from build123d import *

# Parameters (mm, degrees)
F0_R     = 18.9865
F1_DEPTH = 48.6156
F2_R     = 13.97
F3_DEPTH = 23.9141
F4_R     = 10.16
F5_DEPTH = 24.7025
F6_R     = 11.176
F7_DEPTH = 17.78
F8_R     = 14.224
F9_DEPTH = 17.78
F9_TAPER = 13


with BuildPart() as f1:
    # F0 (on Right) → F1 (new body)
    with BuildSketch(Plane.YZ):
        Circle(F0_R)
    extrude(amount=F1_DEPTH)

    # F2 (on face) → F3 (cut)
    with BuildSketch(Plane(origin=(0, 0, 0), x_dir=(0, -1, 0), z_dir=(-1, 0, 0))):
        Circle(F2_R)
    extrude(amount=-F3_DEPTH, mode=Mode.SUBTRACT)

    # F4 (on face) → F5 (cut, through all)
    with BuildSketch(Plane(origin=(23.9141, 0, 0), x_dir=(0, -1, 0), z_dir=(-1, 0, 0))):
        Circle(F4_R)
    extrude(amount=-F5_DEPTH, mode=Mode.SUBTRACT)

    # F6 (on face) → F7 (cut)
    with BuildSketch(Plane.YZ.offset(48.6156)):
        Circle(F6_R)
    extrude(amount=-F7_DEPTH, mode=Mode.SUBTRACT)

    # F8 (on face) → F9 (cut)
    with BuildSketch(Plane.YZ.offset(48.6156)):
        Circle(F8_R)
    extrude(amount=-F9_DEPTH, taper=F9_TAPER, mode=Mode.SUBTRACT)


solid = f1.part
Design review of the part built by this model. Coordinates are the model's own, in mm. A direction names the side the tool comes from. Coordinates: 2 decimals unless noted, no trailing zeros. Loops run counter-clockwise (first coordinate to the right, second up) from the corner with the lowest first, then second, coordinate; pieces in that order, holes last. Notation, with made-up numbers: (-2, 18) -> (30, 18) arc R15 ccw to (30, 23) -> close; hole circle Ø5 at (18.5, -22.5). An arc over 180 degrees is marked (long way). Use a Markdown table: item, result. Add a question column.
Item 1: The part is to be moulded in two halves that separate along Z. For faces 4 (the flat face through (48.616, 2.7, 14.2)), 5 (the cylindrical face through (23.97, 18.11, 5.7)), 6 (the cylindrical face through (33.16, -8.87, -6.8)), say which applies: +Z half, -Z half, draft (parallel to the pull), parting line (faces both ways), or undercut.
Item 2: Machinability: for faces 1 (the cylindrical face through (11.79, 1.82, 13.85)), 2 (the flat face through (0, -10, 10)), 3 (the flat face through (30.836, -3, -10)), which of the approach directions +Z, -Z, +X, -X, +Y, -Y give a long, thin tool a straight path to every point of the face, cutting with its end or side? Answer none if there is none.
Item 3: We need section D-D, the plane x = 38. Write out the cut boundary in (y, z), and give its area (3 significant figures).
Item 4: Wall thickness on L1, parallel to Z at x = 26, y = -0.5; L2, parallel to Z at x = 12, y = 0; L3, parallel to Y at x = 44, z = 11: over which ranges is each line inside the solid? List them lowest first. Write a range as from..to.
Item 5: We need section B-B, the plane x = 8. Write out the cut boundary in (y, z), and give its area (3 significant figures).
Item 6: We need section A-A, the plane y = 0. Write out the cut boundary in (x, z), and give its area (3 significant figures).
Item 7: We need section C-C, the plane z = 16.5. Write out the cut boundary in (x, y).
Item 8: Clearance check with flat-ended pins moving along their axes: P1, Ø14, axis at y = 0, z = 4, coming from the -X side; P2, Ø1.5, axis at x = 16.5, z = -6, coming from the -Y side; P3, Ø10, axis at x = 34, y = 4, coming from the +Z side; P4, Ø12, axis at y = 4, z = -10, coming from the +X side. State where each tip first meets the part, or that it passes through.
Numbers:
| question | item | result |
|---|---|---|
| 1 | face 4 | draft |
| 1 | face 5 | parting line |
| 1 | face 6 | undercut |
| 2 | face 1 | -X |
| 2 | face 2 | +Z, -Z, -X, +Y, -Y |
| 2 | face 3 | +X |
| 3 | outline | circle Ø37.97 at (0, 0); hole circle Ø23.55 at (0, 0) |
| 3 | area | 697 mm^2 |
| 4 | L1 | z = -18.98..-10.15, 10.15..18.98 |
| 4 | L2 | z = -18.99..-13.97, 13.97..18.99 |
| 4 | L3 | y = -15.48..-7.22, 7.22..15.48 |
| 5 | outline | circle Ø37.97 at (0, 0); hole circle Ø27.94 at (0, 0) |
| 5 | area | 519 mm^2 |
| 6 | outline | (0, -18.99) -> (48.62, -18.99) -> (48.62, -14.22) -> (35.41, -11.18) -> (30.84, -11.18) -> (30.84, -10.16) -> (23.91, -10.16) -> (23.91, -13.97) -> (0, -13.97) -> close; (0, 13.97) -> (23.91, 13.97) -> (23.91, 10.16) -> (30.84, 10.16) -> (30.84, 11.18) -> (35.41, 11.18) -> (48.62, 14.22) -> (48.62, 18.99) -> (0, 18.99) -> close |
| 6 | area | 600 mm^2 |
| 7 | outline | (0, -9.39) -> (48.62, -9.39) -> (48.62, 9.39) -> (0, 9.39) -> close |
| 8 | P1 | stops at x = 23.91 |
| 8 | P2 | stops at y = -18.25 |
| 8 | P3 | stops at z = 18.99 |
| 8 | P4 | stops at x = 48.62 |
